from build123d import *

# Parameters (mm, degrees)
PAD_DEPTH            = 6.5
POCKET_DEPTH         = 6
SKETCH002_R          = 13.5
POCKET001_DEPTH      = 1
SKETCH003_W          = 5.4
SKETCH003_H          = 6.5
PAD001_DEPTH         = 4.5
POCKET002_DEPTH      = 10
SKETCH010_W          = 3.95
SKETCH010_H          = 6.5
PAD002_DEPTH         = 4.5
POCKET005_DEPTH      = 10
SKETCH014_R          = 20.45
SKETCH014_R_2        = 19.5
POCKET008_DEPTH      = 0.3
SKETCH015_R          = 2.2
SKETCH015_R_2        = 0.975
PAD003_DEPTH         = 2
POCKET009_DEPTH      = 4
POCKET010_DEPTH      = 4
PAD004_DEPTH         = 4
SKETCH019_R          = 0.6
POCKET011_DEPTH      = 2
SKETCH020_R          = 0.6
POCKET012_DEPTH      = 2
POCKET013_DEPTH      = 12.151
POCKET013_DEPTH_BACK = 36.251


with BuildPart() as part:
    # Sketch → Pad (new body)
    with BuildSketch(Plane.XY):
        with BuildLine():
            Line((-22.5019915649, 16), (-22.5019915649, -16))
            Line((-22.5019915649, -16), (-16.2858834578, -17.9))
            ThreePointArc((-16.2858834578, -17.9), (-0.4552796053, -24.1957169863), (15.6009615088, -18.5))
            Line((15.6009615088, -18.5), (24.5395016581, -17.45))
            Line((24.5395016581, 17.45), (24.5395016581, -17.45))
            Line((15.6009615088, 18.5), (24.5395016581, 17.45))
            ThreePointArc((15.6009615088, 18.5), (-0.4552796053, 24.1957169863), (-16.2858834578, 17.9))
            Line((-22.5019915649, 16), (-16.2858834578, 17.9))
        make_face()
    extrude(amount=PAD_DEPTH)

    # Sketch001 → Pocket (cut)
    with BuildSketch(Plane.XY):
        with BuildLine():
            Line((-14.8539557021, 16.9), (-21.2122180433, 15.55))
            Line((-21.2122180433, 15.55), (-21.2122180433, -15.55))
            Line((-21.2122180433, -15.55), (-14.8539557021, -16.9))
            ThreePointArc((-14.8539557021, -16.9), (-0.0760301383, -22.4998715423), (14.739402973, -17))
            Line((14.739402973, -17), (23.6191552218, -16.4))
            Line((23.6191552218, 16.4), (23.6191552218, -16.4))
            Line((14.739402973, 17), (23.6191552218, 16.4))
            ThreePointArc((14.739402973, 17), (-0.0760301383, 22.4998715423), (-14.8539557021, 16.9))
        make_face()
    extrude(amount=POCKET_DEPTH, mode=Mode.SUBTRACT)

    # Sketch002 (on Face19 of Pocket) → Pocket001 (cut)
    with BuildSketch(Plane(origin=(0, 0, 6), x_dir=(1, 0, 0), z_dir=(0, 0, -1))):
        Circle(SKETCH002_R)
    extrude(amount=-POCKET001_DEPTH, mode=Mode.SUBTRACT)

    # Sketch003 (on Face7 of Pad) → Pad001 (join)
    with BuildSketch(Plane.YZ.offset(24.5395016581)):
        with Locations((-14.75, 3.25)):
            Rectangle(SKETCH003_W, SKETCH003_H)
        with Locations((14.75, 3.25)):
            Rectangle(SKETCH003_W, SKETCH003_H)
    extrude(amount=PAD001_DEPTH)

    # Sketch006 (on Face22 of Pad001) → Pocket002 (cut)
    with BuildSketch(Plane.XY.offset(6.5)):
        with BuildLine():
            ThreePointArc((24.5395016581, 17.45), (26.5735685567, 15.7065020586), (29.0395016581, 14.6594169812))
            Line((29.0395016581, 17.45), (29.0395016581, 14.6594169812))
            Line((29.0395016581, 17.45), (24.5395016581, 17.45))
        make_face()
        with BuildLine():
            ThreePointArc((29.0395016581, -14.6594169811), (26.5735685567, -15.7065020586), (24.5395016581, -17.45))
            Line((29.0395016581, -17.45), (24.5395016581, -17.45))
            Line((29.0395016581, -14.6594169811), (29.0395016581, -17.45))
        make_face()
    extrude(amount=-POCKET002_DEPTH, mode=Mode.SUBTRACT)

    # Sketch010 (on Face3 of Pad) → Pad002 (join)
    with BuildSketch(Plane(origin=(-22.5019915649, 0, 0), x_dir=(0, -1, 0), z_dir=(-1, 0, 0))):
        with Locations((-14.025, 3.25)):
            Rectangle(SKETCH010_W, SKETCH010_H)
        with Locations((14.025, 3.25)):
            Rectangle(SKETCH010_W, SKETCH010_H)
    extrude(amount=PAD002_DEPTH)

    # Sketch011 (on Face28 of Pad002) → Pocket005 (cut)
    with BuildSketch(Plane.XY.offset(6.5)):
        Polygon((-27.0019915649, 16), (-22.5019915649, 16), (-27.0019915649, 14.5), align=None)
        Polygon((-22.5019915649, -16), (-27.0019915649, -14.5), (-27.0019915649, -16), align=None)
    extrude(amount=-POCKET005_DEPTH, mode=Mode.SUBTRACT)

    # Sketch014 (on Face10 of Pad) → Pocket008 (cut)
    with BuildSketch(Plane.XY.offset(6.5)):
        Circle(SKETCH014_R)
        Circle(SKETCH014_R_2, mode=Mode.SUBTRACT)
    extrude(amount=-POCKET008_DEPTH, mode=Mode.SUBTRACT)

    # Sketch015 (on Face19 of Pocket) → Pad003 (join)
    with BuildSketch(Plane(origin=(0, 0, 6), x_dir=(1, 0, 0), z_dir=(0, 0, -1))):
        with Locations((-18.42, 13.32)):
            Circle(SKETCH015_R)
        with Locations((-18.42, 13.32)):
            Circle(SKETCH015_R_2, mode=Mode.SUBTRACT)
        with Locations((7.27, 18.56)):
            Circle(SKETCH015_R)
        with Locations((7.27, 18.56)):
            Circle(SKETCH015_R_2, mode=Mode.SUBTRACT)
        with Locations((5.37, -19.79)):
            Circle(SKETCH015_R)
        with Locations((5.37, -19.79)):
            Circle(SKETCH015_R_2, mode=Mode.SUBTRACT)
        with Locations((-18.42, -13.32)):
            Circle(SKETCH015_R)
        with Locations((-18.42, -13.32)):
            Circle(SKETCH015_R_2, mode=Mode.SUBTRACT)
    extrude(amount=PAD003_DEPTH)

    # Sketch016 → Pocket009 (cut)
    with BuildSketch(Plane(origin=(0, 0, 0), x_dir=(-1, 0, 0), z_dir=(0, 0, 1))):
        with BuildLine():
            Line((-5, 23.6778377391), (-5, 21.9374109685))
            ThreePointArc((5, 21.9374109685), (0, 22.5), (-5, 21.9374109685))
            Line((5, 23.6778377391), (5, 21.9374109685))
            ThreePointArc((5, 23.6778377391), (0, 24.2), (-5, 23.6778377391))
        make_face()
    extrude(amount=POCKET009_DEPTH, mode=Mode.SUBTRACT)

    # Sketch017 → Pocket010 (cut)
    with BuildSketch(Plane(origin=(0, 0, 0), x_dir=(-1, 0, 0), z_dir=(0, 0, 1))):
        with BuildLine():
            Line((-3.499984119, -22.2261132717), (-3.5, -23.9455632634))
            ThreePointArc((-3.5, -23.9455632634), (0, -24.2000019575), (3.5, -23.9455632634))
            Line((3.5000158811, -22.2261082701), (3.5, -23.9455632634))
            ThreePointArc((-3.499984119, -22.2261132717), (1.60767e-05, -22.5), (3.5000158811, -22.2261082701))
        make_face()
        with BuildLine():
            ThreePointArc((-13.9498796389, -17.6536358312), (-11.25, -19.4855715851), (-8.3135572795, -20.9077680626))
            Line((-8.3135572795, -20.9077680626), (-8.9416927184, -22.487466094))
            ThreePointArc((-15.0038705449, -18.987466094), (-12.1, -20.9578147716), (-8.9416927184, -22.487466094))
            Line((-13.9498796389, -17.6536358312), (-15.0038705449, -18.987466094))
        make_face()
        with BuildLine():
            ThreePointArc((8.3135572795, -20.9077680626), (11.25, -19.4855715851), (13.9498796389, -17.6536358312))
            Line((13.9498796389, -17.6536358312), (15.0038705449, -18.987466094))
            ThreePointArc((8.9416927184, -22.487466094), (12.1, -20.9578147716), (15.0038705449, -18.987466094))
            Line((8.3135572795, -20.9077680626), (8.9416927184, -22.487466094))
        make_face()
    extrude(amount=POCKET010_DEPTH, mode=Mode.SUBTRACT)

    # Sketch018 (on Face8 of Pocket005) → Pad004 (join)
    with BuildSketch(Plane(origin=(0, 0, 0), x_dir=(1, 0, 0), z_dir=(0, 0, -1))):
        Polygon((-27.0019915649, 14.5), (-27.0019915649, 12.05), (-22.5019915649, 12.05), (-22.5019915649, 16), align=None)
        Polygon((-27.0019915649, -12.05), (-22.5019915649, -12.05), (-22.5019915649, -16), (-27.0019915649, -14.5), align=None)
        with BuildLine():
            Line((24.5395016581, 17.45), (24.5395016581, 12.05))
            Line((29.0395016581, 12.05), (24.5395016581, 12.05))
            Line((29.0395016581, 14.6594169811), (29.0395016581, 12.05))
            ThreePointArc((24.5395016581, 17.45), (26.5735685567, 15.7065020586), (29.0395016581, 14.6594169811))
        make_face()
        with BuildLine():
            Line((24.5395016581, -12.05), (24.5395016581, -17.45))
            ThreePointArc((29.0395016581, -14.6594169811), (26.5735685568, -15.7065020586), (24.5395016581, -17.45))
            Line((29.0395016581, -12.05), (29.0395016581, -14.6594169812))
            Line((24.5395016581, -12.05), (29.0395016581, -12.05))
        make_face()
    extrude(amount=PAD004_DEPTH)

    # Sketch019 (on Face64 of Pad004) → Pocket011 (cut)
    with BuildSketch(Plane.XZ.offset(-12.05)):
        with Locations((27.7395016581, -2.7)):
            Circle(SKETCH019_R)
        with Locations((-25.7019915649, -2.7)):
            Circle(SKETCH019_R)
    extrude(amount=-POCKET011_DEPTH, mode=Mode.SUBTRACT)

    # Sketch020 (on Face50 of Pocket011) → Pocket012 (cut)
    with BuildSketch(Plane(origin=(0, -12.05, 0), x_dir=(-1, 0, 0), z_dir=(0, 1, 0))):
        with Locations((-27.7395016581, -2.7)):
            Circle(SKETCH020_R)
        with Locations((25.7019915649, -2.7)):
            Circle(SKETCH020_R)
    extrude(amount=-POCKET012_DEPTH, mode=Mode.SUBTRACT)

    # Sketch021 (on Face48 of Pocket012) → Pocket013 (cut, two sides)
    with BuildSketch(Plane.XZ.offset(-12.05)) as pocket013_sk:
        with BuildLine():
            ThreePointArc((29.0395016581, 0), (27.8047252112, 3.9528470752), (24.5395016581, 6.5))
            Line((24.5395016581, 6.5), (29.0395016581, 6.5))
            Line((29.0395016581, 6.5), (29.0395016581, 0))
        make_face()
        with BuildLine():
            ThreePointArc((24.5395016581, -1.478433716), (25.560340141, -3.0916708473), (27.2395016581, -4))
            Line((24.5395016581, -4), (27.2395016581, -4))
            Line((24.5395016581, -1.478433716), (24.5395016581, -4))
        make_face()
        with BuildLine():
            ThreePointArc((-22.5019915649, 6.5), (-25.767215118, 3.9528470752), (-27.0019915649, 0))
            Line((-27.0019915649, 6.5), (-27.0019915649, 0))
            Line((-22.5019915649, 6.5), (-27.0019915649, 6.5))
        make_face()
        with BuildLine():
            ThreePointArc((-25.3019915649, -4), (-23.3759624024, -3.1260291625), (-22.5019915649, -1.2))
            Line((-22.5019915649, -1.2), (-22.5019915649, -4))
            Line((-22.5019915649, -4), (-25.3019915649, -4))
        make_face()
    extrude(amount=-POCKET013_DEPTH, mode=Mode.SUBTRACT)
    extrude(pocket013_sk.sketch, amount=POCKET013_DEPTH_BACK, mode=Mode.SUBTRACT)


solid = part.part
Geometry: final body of the model. Coordinates: model frame, mm. A direction names the side the tool comes from. Coordinates: 2 decimals unless noted, no trailing zeros. Loops run counter-clockwise (first coordinate to the right, second up) from the corner with the lowest first, then second, coordinate; pieces in that order, holes last. Notation, with made-up numbers: M -19,-35 L 25,-35 A27 cw 25,0 Z; hole C 64.25,86.25 d2. An arc over 180 degrees is marked long. One line per item, written item: value. Start each with the question number.
1) Cut plane D-D (y = -4). Return loops of the section in (x, z), then the cut area to 3 significant figures.
2) Pin query (flat end, axial travel): P1, Ø2, axis at x = 27.5, z = 0.5, coming from the -Y side; P2, Ø1.3, axis at x = 5.5, y = 19, coming from the -Z side; P3, Ø2.5, axis at x = 5, y = 22.5, coming from the -Z side; P4, Ø3, axis at x = 0.5, z = 2, coming from the -Y side. Return the tip coordinate at first contact, or that it passes through.
3) Cut plane A-A (y = 10). Return loops of the section in (x, z).
4) Reachability of faces 1 (the cylindrical face through (-25.148, 13.036, -2.93)), 2 (the flat face through (-14.47, 18.31, 1.97)), 3 (the flat face through (-8.623, 21.687, 1.972)), 4 (the cylindrical face through (4.596, 20.383, 5.014)) from +Z, -Z, +X, -X, +Y, -Y: full face, straight path, thin tool, end or side. Return the list, or none.
5) Draft query along X for faces 5 (the flat face through (19.117, -16.704, 2.958)), 6 (the cylindrical face through (-25.733, 13.558, 4.001)), 7 (the flat face through (11, -10, 6)), 8 (the flat face through (28, -13, -4)). Return one class per face: released by +X, released by -X, zero draft, split by the parting line, or undercut.
6) Material intervals for L1, parallel to Y at x = 0, z = 6.3; L2, parallel to X at y = 13.32, z = 4.95 (3 decimals); L3, parallel to X at y = -13.32, z = 5.5 (3 decimals), sorted ascending. Write a range as from..to.
7) Cut plane B-B (z = -2.7). Count the separate pieces of the cut face and the enclosed holes in it, then the cut area to 3 significant figures.
Evaluation:
1. outline: M -22.5,0 L -21.21,0 L -21.21,6 L -12.89,6 L -12.89,6.5 L -19.09,6.5 L -19.09,6.2 L -20.05,6.2 L -20.05,6.5 L -22.5,6.5 Z; M 12.89,6 L 23.62,6 L 23.62,0 L 24.54,0 L 24.54,6.5 L 20.05,6.5 L 20.05,6.2 L 19.09,6.2 L 19.09,6.5 L 12.89,6.5 Z
1. area: 23.3 mm^2
2. P1: y = -15.75
2. P2: z = 4
2. P3: z = 0
2. P4: through
3. outline: M -22.5,0 L -21.21,0 L -21.21,6 L -9.07,6 L -9.07,6.5 L -16.74,6.5 L -16.74,6.2 L -17.84,6.2 L -17.84,6.5 L -22.5,6.5 Z; M 9.07,6 L 23.62,6 L 23.62,0 L 24.54,0 L 24.54,6.5 L 17.84,6.5 L 17.84,6.2 L 16.74,6.2 L 16.74,6.5 L 9.07,6.5 Z
4. face 1: none
4. face 2: -Z, +Y
4. face 3: -Z, -X
4. face 4: -Z
5. face 5: undercut
5. face 6: released by -X
5. face 7: undercut
5. face 8: zero draft
6. L1: -24.2..-20.45, -19.5..-13.5, 13.5..19.5, 20.45..24.2
6. L2: -24.928..-21.212, -20.62..-19.395, -17.445..-16.22, 23.619..26.966
6. L3: -24.297..-21.212, -20.62..-19.395, -17.445..-16.22, 23.619..26.335
7. separate pieces: 4
7. enclosed holes: 0
7. area: 41.7 mm^2
